Check sheet for the modelled part. Datum: model origin and axes. Units: mm. A direction names the side the tool comes from. Give positions to 0.01 mm unless a question says otherwise; leave off trailing zeros. Loops run counter-clockwise (first coordinate to the right, second up) from the corner with the lowest first, then second, coordinate; pieces in that order, holes last. Notation, with made-up numbers: (43, 0) - (57, 0) arc R20 cw to (57, 37) - close; hole circle Ø6 at (-9, 32). An arc over 180 degrees is marked (long way). Use CSV: the item, a comma, the result in double quotes.
from build123d import *

# Parameters (mm, degrees)
BOSS_EXTRUDE1_DEPTH         = 22.225
F_1_4_20_TAPPED_HOLE1_D     = 5.1054
F_1_4_20_TAPPED_HOLE1_DEPTH = 12.7
F_1_4_20_TAPPED_HOLE1_TIP   = 1.533816902
FILLET1_R                   = 3.175


with BuildPart() as part:
    # Sketch1 → Boss-Extrude1 (new body)
    with BuildSketch(Plane(origin=(0, 0, 0), x_dir=(1, 0, 0), z_dir=(0, 1, 0))):
        with BuildLine():
            Line((50.8, 3.175), (50.8, -3.175))
            ThreePointArc((50.8, -3.175), (0, -53.975), (-50.8, -3.175))
            Line((-50.8, -3.175), (-50.8, 3.175))
            ThreePointArc((-50.8, 3.175), (0, 53.975), (50.8, 3.175))
        make_face()
    extrude(amount=BOSS_EXTRUDE1_DEPTH)

    # 1/4-20 Tapped Hole1
    with Locations(Plane(origin=(0, 22.225, 0), x_dir=(1, 0, 0), z_dir=(0, 1, 0))):
        with Locations((-24.99995, 24.99995), (24.99995, 24.99995), (24.99995, -24.99995), (-24.99995, -24.99995)):
            Hole(F_1_4_20_TAPPED_HOLE1_D / 2, depth=F_1_4_20_TAPPED_HOLE1_DEPTH)
            with Locations((0, 0, -(F_1_4_20_TAPPED_HOLE1_DEPTH + F_1_4_20_TAPPED_HOLE1_TIP / 2))):  # 118° drill point
                Cone(0, F_1_4_20_TAPPED_HOLE1_D / 2, F_1_4_20_TAPPED_HOLE1_TIP, mode=Mode.SUBTRACT)

    # Fillet1
    fillet1_edges = [part.edges().sort_by_distance(p)[0] for p in [
        (0, 22.225, 53.975),
        (50.8, 22.225, 0),
        (0, 22.225, -53.975),
        (-50.8, 22.225, 0),
    ]]
    fillet(fillet1_edges, radius=FILLET1_R)


solid = part.part
1. Go/stop test with flat-tipped pins: pin 1 Ø2 at (y, z) = (19, 33) entering from +X; pin 2 Ø3 at (x, z) = (25, -25) entering from +Y; pin 3 Ø3 at (x, y) = (15, 3.5) entering from -Z. Record where each tip stops, or that it passes through.
Completed:
pin 1,"stops at x = 41.83"
pin 2,"stops at y = 8.89"
pin 3,"stops at z = -52.15"
2. Set-up check for faces 1 (the face through (25.33, 15.79, 22.47)), 2 (the face through (50.8, 9, 0)): record each of +Z, -Z, +X, -X, +Y, -Y from which the full face is reachable in a straight line by a thin tool's end or side.
Completed:
face 1,"+Y"
face 2,"+Z, -Z, +X, +Y, -Y"
3. Scan lines: line 1 along Z through (x, y) = (-23, 17); line 2 along Z through (x, y) = (40, 1.75); line 3 along X through (y, z) = (1.75, -48.5). Record each from-to range of solid material in increasing order.
Completed:
line 1,"z = -48.47 to -26.59, -23.41 to 23.41, 26.59 to 48.47"
line 2,"z = -34.49 to 34.49"
line 3,"x = -22.94 to 22.94"
4. Sectioned sample at A-A, the plane y = 16.75. Record the boundary of the cut face in (x, z) (3 decimals).
Completed:
outline,"(-50.8, -3.175) arc R50.8 ccw to (50.8, -3.175) - (50.8, 3.175) arc R50.8 ccw to (-50.8, 3.175) - close; hole circle Ø5.105 at (-25, -25); hole circle Ø5.105 at (-25, 25); hole circle Ø5.105 at (25, -25); hole circle Ø5.105 at (25, 25)"
5. Release check for a two-part mould opening along Z. For faces 3 (the face through (-23.119, 15.786, -26.725)), 4 (the face through (49.895, 21.27, 0.044)), 5 (the face through (-1.117, 9.392, -53.963)), 6 (the face through (24.94, 8.26, -25.44)) record: released by +Z, released by -Z, zero draft, split by the parting line, or undercut.
Completed:
face 3,"undercut"
face 4,"zero draft"
face 5,"released by -Z"
face 6,"undercut"
6. Sectioned sample at B-B, the plane y = 3.5. Record the boundary of the cut face in (x, z) (3 decimals).
Completed:
outline,"(-50.8, -3.175) arc R50.8 ccw to (50.8, -3.175) - (50.8, 3.175) arc R50.8 ccw to (-50.8, 3.175) - close"
